CAD build for the part. Positions are in the model's coordinates, mm. A direction names the side the tool comes from. Give positions to 0.01 mm unless a question says otherwise; leave off trailing zeros. Write each loop counter-clockwise with the first axis right and the second up, starting at its lowest first coordinate (ties: lowest second). Pieces come first, ordered by that corner, then holes. Notation, with made-up numbers: (-37, 19.25) - (18, 19.25) arc R25 cw to (18, 47.25) - close; hole circle Ø11 at (-21.5, 81.5). An arc over 180 degrees is marked (long way). Answer as a JSON object with one key per item and string values.
from build123d import *

# Parameters (mm, degrees)
F1_DEPTH = 33
F2_W     = 210
F2_H     = 126
F3_DEPTH = 3
F4_W     = 40
F4_H     = 10
F5_DEPTH = 210.001
F6_R     = 5
F7_R     = 3
F8_DEPTH = 20


with BuildPart() as f1:
    # F0 (on Top) → F1 (new body)
    with BuildSketch(Plane.XY):
        with BuildLine():
            Line((105, 57), (105, 63))
            Line((105, 63), (99, 63))
            ThreePointArc((99, 63), (103.2426406871, 61.2426406871), (105, 57))
        make_face()
        with BuildLine():
            ThreePointArc((-105, 57), (-103.2426406871, 61.2426406871), (-99, 63))
            Line((-99, 63), (-105, 63))
            Line((-105, 63), (-105, 57))
        make_face()
        with BuildLine():
            Line((105, -63), (105, -57))
            ThreePointArc((105, -57), (103.2426406871, -61.2426406871), (99, -63))
            Line((99, -63), (105, -63))
        make_face()
        with BuildLine():
            ThreePointArc((-99, -63), (-103.242640668, -61.2426407063), (-105, -57.0000000541))
            Line((-105, -57.0000000541), (-105, -63))
            Line((-105, -63), (-99, -63))
        make_face()
        with BuildLine():
            Line((-99, -63), (99, -63))
            ThreePointArc((99, -63), (95.5358983849, -61.8989794856), (93.3431457505, -59))
            Line((93.3431457505, -59), (-93.3431457505, -59))
            ThreePointArc((-93.3431457505, -59), (-95.5358983849, -61.8989794856), (-99, -63))
        make_face()
        with BuildLine():
            Line((105, -57), (105, 57))
            ThreePointArc((105, 57), (103.8989794856, 53.5358983849), (101, 51.3431457505))
            Line((101, 51.3431457505), (101, -51.3431457505))
            ThreePointArc((101, -51.3431457505), (103.8989794856, -53.5358983849), (105, -57))
        make_face()
        with BuildLine():
            ThreePointArc((-101, 51.3431457505), (-103.8989794856, 53.5358983849), (-105, 57))
            Line((-105, 57), (-105, -57.0000000541))
            ThreePointArc((-105, -57.0000000541), (-103.8989795012, -53.535898407), (-101, -51.3431457505))
            Line((-101, -51.3431457505), (-101, 51.3431457505))
        make_face()
        with BuildLine():
            ThreePointArc((-93.3431457505, 59), (-95.5358983849, 61.8989794856), (-99, 63))
            ThreePointArc((-99, 63), (-103.2426406871, 61.2426406871), (-105, 57))
            ThreePointArc((-105, 57), (-103.8989794856, 53.5358983849), (-101, 51.3431457505))
            Line((-101, 51.3431457505), (-101, 59))
            Line((-101, 59), (-93.3431457505, 59))
        make_face()
        with BuildLine():
            ThreePointArc((-101, -51.3431457505), (-103.8989795012, -53.535898407), (-105, -57.0000000541))
            ThreePointArc((-105, -57.0000000541), (-103.242640668, -61.2426407063), (-99, -63))
            ThreePointArc((-99, -63), (-95.5358983849, -61.8989794856), (-93.3431457505, -59))
            Line((-93.3431457505, -59), (-101, -59))
            Line((-101, -59), (-101, -51.3431457505))
        make_face()
        with BuildLine():
            ThreePointArc((105, 57), (103.2426406871, 61.2426406871), (99, 63))
            ThreePointArc((99, 63), (95.5358983849, 61.8989794856), (93.3431457505, 59))
            Line((93.3431457505, 59), (101, 59))
            Line((101, 59), (101, 51.3431457505))
            ThreePointArc((101, 51.3431457505), (103.8989794856, 53.5358983849), (105, 57))
        make_face()
        with BuildLine():
            ThreePointArc((99, -63), (103.2426406871, -61.2426406871), (105, -57))
            ThreePointArc((105, -57), (103.8989794856, -53.5358983849), (101, -51.3431457505))
            Line((101, -51.3431457505), (101, -59))
            Line((101, -59), (93.3431457505, -59))
            ThreePointArc((93.3431457505, -59), (95.5358983849, -61.8989794856), (99, -63))
        make_face()
        with BuildLine():
            Line((101, 59), (93.3431457505, 59))
            ThreePointArc((93.3431457505, 59), (94.7573593129, 52.7573593129), (101, 51.3431457505))
            Line((101, 51.3431457505), (101, 59))
        make_face()
        with BuildLine():
            ThreePointArc((-93, 57), (-93.0864086421, 58.0146118724), (-93.3431457505, 59))
            Line((-93.3431457505, 59), (-101, 59))
            Line((-101, 59), (-101, 51.3431457505))
            ThreePointArc((-101, 51.3431457505), (-95.5358983849, 52.1010205144), (-93, 57))
        make_face()
        with BuildLine():
            ThreePointArc((-93, -57), (-95.5358983849, -52.1010205144), (-101, -51.3431457505))
            Line((-101, -51.3431457505), (-101, -59))
            Line((-101, -59), (-93.3431457505, -59))
            ThreePointArc((-93.3431457505, -59), (-93.0864086421, -58.0146118724), (-93, -57))
        make_face()
        with BuildLine():
            Line((101, -59), (101, -51.3431457505))
            ThreePointArc((101, -51.3431457505), (94.7573593129, -52.7573593129), (93.3431457505, -59))
            Line((93.3431457505, -59), (101, -59))
        make_face()
        with BuildLine():
            ThreePointArc((93.3431457505, 59), (95.5358983849, 61.8989794856), (99, 63))
            Line((99, 63), (-99, 63))
            ThreePointArc((-99, 63), (-95.5358983849, 61.8989794856), (-93.3431457505, 59))
            Line((-93.3431457505, 59), (93.3431457505, 59))
        make_face()
    extrude(amount=F1_DEPTH)

    # F2 (on Top) → F3 (join)
    with BuildSketch(Plane.XY):
        Rectangle(F2_W, F2_H)
    extrude(amount=F3_DEPTH)

    # F4 (on face) → F5 (cut, through all)
    with BuildSketch(Plane.YZ.offset(105)):
        with Locations((0, 9)):
            Rectangle(F4_W, F4_H)
    extrude(amount=-F5_DEPTH, mode=Mode.SUBTRACT)

    # F6
    f6_edges = [f1.edges().sort_by_distance(p)[0] for p in [
        (-105, 63, 16.5),
        (105, 63, 16.5),
        (105, -63, 16.5),
        (-105, -63, 16.5),
    ]]
    fillet(f6_edges, radius=F6_R)

    # F7 (on face) → F8 (cut)
    with BuildSketch(Plane.XY.offset(33)):
        with Locations((-99, 57)):
            Circle(F7_R)
        with Locations((99, 57)):
            Circle(F7_R)
        with Locations((99, -57)):
            Circle(F7_R)
        with Locations((-99, -57)):
            Circle(F7_R)
    extrude(amount=-F8_DEPTH, mode=Mode.SUBTRACT)


solid = f1.part
Item 1: Cut at A-A (z = 25). Give the cut face in (x, y), and give its area (3 significant figures).
Entries:
{"outline": "(-105, -58) arc R5 ccw to (-100, -63) - (100, -63) arc R5 ccw to (105, -58) - (105, 58) arc R5 ccw to (100, 63) - (-100, 63) arc R5 ccw to (-105, 58) - close; hole circle Ø6 at (-99, -57); hole circle Ø6 at (-99, 57); hole (-101, -51.34) arc R6 cw to (-93.34, -59) - (93.34, -59) arc R6 cw to (101, -51.34) - (101, 51.34) arc R6 cw to (93.34, 59) - (-93.34, 59) arc R6 cw to (-101, 51.34) - close; hole circle Ø6 at (99, -57); hole circle Ø6 at (99, 57)", "area": "2,710 mm2"}
Item 2: Cut at C-C (x = 79.5). Give the cut face in (y, z), and give its area (3 significant figures).
Entries:
{"outline": "(-63, 0) - (63, 0) - (63, 33) - (59, 33) - (59, 3) - (-59, 3) - (-59, 33) - (-63, 33) - close", "area": "618 mm2"}
Item 3: Mould opens along Y. For faces 4 (the flat face through (1, -59, 18)), 5 (the flat face through (-1, -63, 16)), 6 (the cylindrical face through (-103, 62, 17)), 7 (the flat face through (-32, 61, 33)) say: +Y half, -Y half, draft (parallel to the pull), parting line (faces both ways), or undercut.
Entries:
{"face 4": "undercut", "face 5": "-Y half", "face 6": "+Y half", "face 7": "draft"}
Item 4: Cut at B-B (y = -38.5). Give the cut face in (x, z).
Entries:
{"outline": "(-105, 0) - (105, 0) - (105, 33) - (101, 33) - (101, 3) - (-101, 3) - (-101, 33) - (-105, 33) - close"}
Item 5: Probe line 1 (Y direction, x = 99, z = 22); line 2 (Y direction, x = -40, z = 19); line 3 (X direction, y = -22.5, z = 13). List the from-to ranges inside material, lowest first. Write a range as from..to.
Entries:
{"line 1": "-63..-60, -54..-51, 51..54, 60..63", "line 2": "-63..-59, 59..63", "line 3": "-105..-101, 101..105"}
Item 6: Which spindle directions (+Z, -Z, +X, -X, +Y, -Y) get a long thin tool onto all of the face, cutting with end or side? Do faces 1 (the cylindrical face through (104, -61, 16)), 2 (the flat face through (-1, 59, 18)), 3 (the flat face through (-103, 20, 9)). Say none if no direction does.
Entries:
{"face 1": "+Z, -Z, +X, -Y", "face 2": "+Z", "face 3": "+X, -X"}
Item 7: Flat gauge pins, fed straight in: P1, Ø3, axis at x = -98, y = -56.5, coming from the +Z side; P2, Ø3, axis at x = -102.5, z = 11, coming from the -Y side; P3, Ø5, axis at x = -21.5, y = 27, coming from the +Z side. Where does each tip first touch, or does it go through?
Entries:
{"P1": "z = 13", "P2": "y = -62.9", "P3": "z = 3"}
